from build123d import *

# Parameters (mm, degrees)
LOFT1_DEPTH        = 508
LOFT1_TAPER        = -7.093868
SHELL1_T           = -19.05
SKETCH5_R          = 147.867108762
CUT_EXTRUDE1_DEPTH = 20
CUT_EXTRUDE2_DEPTH = 526.768458633
CUT_EXTRUDE2_TAPER = -20
CIRPATTERN1_COUNT  = 18


# Read off the part's stored shape, not the designer's step: Loft1
with BuildPart() as part:
    # Loft1 outline → Loft1 (new body)
    with BuildSketch(Plane(origin=(0, -508, 0), x_dir=(1, 0, 0), z_dir=(0, 1, 0))):
        Polygon((31.896938478, -55.24711805), (48.868944947, -41.005913681), (59.946635427, -21.81879094), (63.793876956, 0), (59.946635427, 21.81879094), (48.868944947, 41.005913681), (31.896938478, 55.24711805), (11.07769048, 62.824704621), (-11.07769048, 62.824704621), (-31.896938478, 55.24711805), (-48.868944947, 41.005913681), (-59.946635427, 21.81879094), (-63.793876956, 0), (-59.946635427, -21.81879094), (-48.868944947, -41.005913681), (-31.896938478, -55.24711805), (-11.07769048, -62.824704621), (11.07769048, -62.824704621), align=None)
    extrude(amount=LOFT1_DEPTH, taper=LOFT1_TAPER)

    # Shell1
    shell1_openings = [part.faces().sort_by_distance(p)[0] for p in [
        (0, 0, 0),
    ]]
    offset(amount=SHELL1_T, openings=shell1_openings, kind=Kind.INTERSECTION)

    # Sketch5 → Cut-Extrude1 (cut)
    with BuildSketch(Plane.XZ.offset(508)):
        Circle(SKETCH5_R)
    extrude(amount=-CUT_EXTRUDE1_DEPTH, mode=Mode.SUBTRACT)

    # Sketch6 → Cut-Extrude2 (cut, through all)
    with BuildSketch(Plane(origin=(-57.914835054, -472.553286642, -10.211948003), x_dir=(0.173648177666931, 0, -0.984807753012208), z_dir=(-0.12161910183404463, -0.9923451605496023, -0.021444729022872505))):
        Polygon((-11.516560933, 125.079390032), (-8.131620777, 106.029390032), (8.131620777, 106.029390032), (11.516560933, 125.079390032), align=None)
    cut_extrude2 = extrude(amount=CUT_EXTRUDE2_DEPTH, taper=CUT_EXTRUDE2_TAPER, mode=Mode.SUBTRACT)

    # CirPattern1: Cut-Extrude2 ×18 about axis
    cirpattern1_axis = Axis((0, 0, 0), (0, 1, 0))
    for i in range(1, CIRPATTERN1_COUNT):
        add(cut_extrude2.rotate(cirpattern1_axis, i * 360 / CIRPATTERN1_COUNT), mode=Mode.SUBTRACT)


solid = part.part
Build history of the part. All positions in model axes, mm. Give positions to 0.01 mm unless a question says otherwise; leave off trailing zeros. Use one line per item in the form item = value.
1) Drop flat-ended pins along their axis: pin 1 (5 mm diameter, centred on y = -234.5, z = -18.5, fed in from +X); pin 2 (2 mm diameter, centred on y = -60, z = 73, fed in from -X); pin 3 (10 mm diameter, centred on x = 51.5, y = -120, fed in from +Z). Give the stop position or say it passes through.
Calculated:
pin_1 = 95.64
pin_2 = -95.37
pin_3 = 101.43
2) Probe probe 1 along X at (y, z) = (-414, -30); probe 2 along Z at (x, y) = (-72.5, -115.5); probe 3 along Z at (x, y) = (46.5, -332.5). List the from-to ranges inside material, lowest first.
Calculated:
probe_1 = -68.73 to -46.56, 46.56 to 68.73
probe_2 = -84.94 to -59.37, 59.37 to 84.94
probe_3 = -71.5 to -46.44, 46.44 to 71.5
3) Two-plate mould, pull along Z, no slides. Class faces 1 (the face through (-19.825, -487.066, 54.303)), 2 (the face through (-72.67, -185.51, 41.65)), 3 (the face through (40.4, 0, -99.3)): released by +Z, released by -Z, zero draft, split by the parting line, or undercut.
Calculated:
face_1 = undercut
face_2 = undercut
face_3 = zero draft
